Source: CAD feature listing. Evaluate the final solid. Frame: model axes, mm. Face numbers are marked on the shaded views. A direction names the side the tool comes from. Give positions to 0.01 mm unless a question says otherwise; leave off trailing zeros. Order: outer loops, then holes, each group sorted by start corner. A loop starts at its lowest first (then second) coordinate and runs counter-clockwise, first axis right, second up. Notation, with made-up numbers: M 68.5,-28.5 L 94.5,-28.5 A23 cw 94.5,-10.5 Z; hole C 50.5,68 d11. An arc over 180 degrees is marked long. One line per question, with ' | ' between items. Start each with the question number.
from build123d import *

# Parameters (mm, degrees)
F0_R     = 25
F1_DEPTH = 88
F3_DEPTH = 50
F5_DEPTH = 16
F6_R     = 6
F7_DEPTH = 9.001572688


with BuildPart() as f1:
    # F0 (on Top) → F1 (new body)
    with BuildSketch(Plane.XY):
        with BuildLine():
            Line((0, 75), (0, 0))
            Line((0, 0), (50, 0))
            ThreePointArc((50, 0), (12.5, 37.5), (50, 75))
            Line((50, 75), (0, 75))
        make_face()
        with BuildLine():
            ThreePointArc((50, 75), (12.5, 37.5), (50, 0))
            ThreePointArc((50, 0), (76.5165042945, 10.9834957055), (87.5, 37.5))
            ThreePointArc((87.5, 37.5), (76.5165042945, 64.0165042945), (50, 75))
        make_face()
        with Locations((50, 37.5)):
            Circle(F0_R, mode=Mode.SUBTRACT)
    extrude(amount=F1_DEPTH)

    # F2 (on Right) → F3 (join)
    with BuildSketch(Plane.YZ):
        Polygon((-88, 0), (0, 0), (0, 20), (0, 40), (-88, 40), align=None)
        with BuildLine():
            ThreePointArc((-25.000251984, 30.9999999971), (-17.2219144973, 27.7782636823), (-14, 20))
            ThreePointArc((-14, 20), (-17.2241933288, 12.2194582058), (-25.0066964749, 9.0000020383))
            Line((-25.0066964749, 9.0000020383), (-62.293662929, 9.0227012457))
            ThreePointArc((-62.293662929, 9.0227012457), (-63.0066964749, 9.0000020383), (-63.7197018551, 9.0235693762))
            ThreePointArc((-63.7197018551, 9.0235693762), (-73.9961566797, 20.2907546668), (-63.1386355855, 30.9991263369))
            ThreePointArc((-63.1386355855, 30.9991263369), (-63.000251984, 30.9999999971), (-62.8618683426, 30.999132677))
            Line((-62.8618683426, 30.999132677), (-25.000251984, 30.9999999971))
        make_face(mode=Mode.SUBTRACT)
    extrude(amount=F3_DEPTH)

    # F4 (on Right) → F5 (join)
    with BuildSketch(Plane.YZ):
        Polygon((-88, 40), (0, 40), (0, 88), align=None)
    extrude(amount=F5_DEPTH)

    # F6 (on face) → F7 (cut, through all)
    with BuildSketch(Plane.XY.offset(40)):
        with Locations((33, -44)):
            Circle(F6_R)
    extrude(amount=-F7_DEPTH, mode=Mode.SUBTRACT)


solid = f1.part
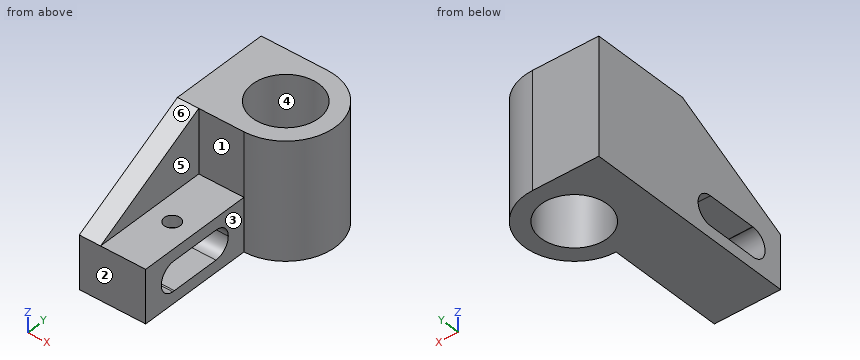
Item 1: Cut plane C-C on y = 19. Return the cut outline in (x, z).
Item 2: Line query: line 1 (X direction, y = -44, z = 36.5); line 2 (Y direction, x = 33, z = 34); line 3 (Y direction, x = 50, z = 65). Output: solid intervals per line, ascending.
Item 3: Pin query (flat end, axial travel): pin 1 Ø1.5 at (x, z) = (70, 23.5) entering from -Y; pin 2 Ø17 at (x, y) = (36.5, -49.5) entering from +Z; pin 3 Ø8 at (y, z) = (8, 52.5) entering from +X. Return the tip coordinate at first contact, or that it passes through.
Item 4: Mould query, pull axis Y, two halves, no side actions, for the marked faces 4, 5 and 6. Classes: pulls with the +Y half, pulls with the -Y half, needs draft (parallel to the pull), parting line crosses it, or undercut.
Item 5: Cut plane D-D on x = 48. Return the cut outline in (y, z), and give its area (3 significant figures).
Item 6: Reachability of the marked faces 1, 2 and 3 from +Z, -Z, +X, -X, +Y, -Y: full face, straight path, thin tool, end or side. Return the list, or none.
Item 7: Cut plane B-B on z = 53.5. Return the cut outline in (x, y).
Item 8: Cut plane A-A on x = 18.5. Return the cut outline in (y, z).
Results are:
1) outline: M 0,0 L 33.18,0 L 33.18,88 L 0,88 Z; M 66.82,0 L 82.62,0 L 82.62,88 L 66.82,88 Z
2) line 1: x = 0 to 27, 39 to 50 | line 2: y = -88 to -50, -38 to 19.17, 55.83 to 75 | line 3: y = 0 to 12.5, 62.5 to 75
3) pin 1: stops at y = 5.32 | pin 2: stops at z = 40 | pin 3: stops at x = 77.5
4) face 4: undercut | face 5: needs draft | face 6: pulls with the -Y half
5) outline: M -88,0 L 12.58,0 L 12.58,88 L 0,88 L 0,40 L -88,40 Z; M 62.42,0 L 75,0 L 75,88 L 62.42,88 Z; hole M -62.86,31 A11 ccw long -62.29,9.02 L -25.01,9 A11 ccw -25,31 Z | area: 4,520 mm2
6) face 1: +Z, +X, -Y | face 2: +Z, -Z, +X, -X, -Y | face 3: +Z, -Z, +X, -Y
7) outline: M 0,-63.25 L 16,-63.25 L 16,0 L 50,0 A37.5 ccw 50,75 L 0,75 Z; hole C 50,37.5 d50
8) outline: M -88,0 L 75,0 L 75,88 L 0,88 L 0,40 L -88,40 Z; hole M -62.86,31 A11 ccw long -62.29,9.02 L -25.01,9 A11 ccw -25,31 Z
